The model under review builds one solid part; all positions refer to its coordinate system, in mm. Face numbers are marked on the shaded views. A direction names the side the tool comes from. Coordinates: 2 decimals unless noted, no trailing zeros. Loops run counter-clockwise (first coordinate to the right, second up) from the corner with the lowest first, then second, coordinate; pieces in that order, holes last. Notation, with made-up numbers: M 23,6 L 40,6 A20 cw 40,21 Z; hole C 28,-21.75 d1. An arc over 180 degrees is marked long. Return JSON: item names as keys, results as strings.
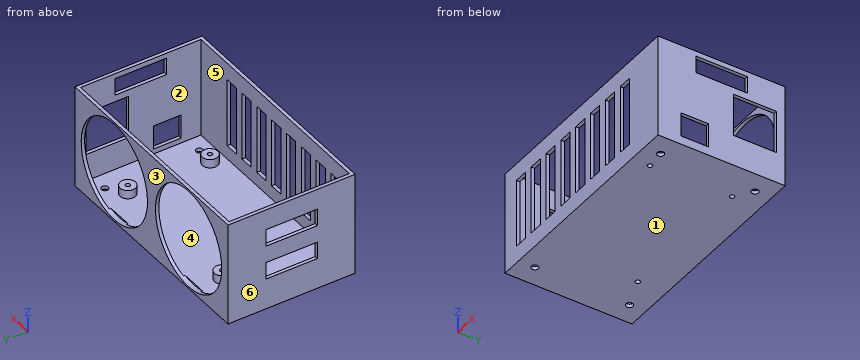
```python
from build123d import *
from build123d.topology import SkipClean

# Parameters (mm, degrees)
ESBO_O1_W                = 134
ESBO_O1_H                = 74
ESBO_O1_W_2              = 130
ESBO_O1_H_2              = 70
RESSALTO_EXTRUS_O1_DEPTH = 60
ESBO_O2_W                = 134
ESBO_O2_H                = 74
ESBO_O2_R                = 2
RESSALTO_EXTRUS_O2_DEPTH = 2
ESBO_O3_W                = 25
ESBO_O3_H                = 25
ESBO_O3_W_2              = 14
ESBO_O3_H_2              = 16
ESBO_O3_W_3              = 10
ESBO_O3_H_3              = 30
CORTE_EXTRUS_O1_DEPTH    = 10
ESBO_O6_W                = 8
ESBO_O6_H                = 40
CORTE_EXTRUS_O2_DEPTH    = 10
ESBO_O7_W                = 10
ESBO_O7_H                = 30
CORTE_EXTRUS_O3_DEPTH    = 12
ESBO_O8_R                = 4.5
ESBO_O8_R_2              = 1.35
RESSALTO_EXTRUS_O3_DEPTH = 5
ESBO_O8_3_R              = 1.35
CORTE_EXTRUS_O4_DEPTH    = 97.031244915
ESBO_O9_R                = 3
CORTE_EXTRUS_O5_DEPTH    = 2
ESBO_O10_R               = 29
CORTE_EXTRUS_O6_DEPTH    = 3


with BuildPart() as part:
    # Esboço1 → Ressalto-extrusão1 (new body)
    with BuildSketch(Plane.XY):
        Rectangle(ESBO_O1_W, ESBO_O1_H)
        Rectangle(ESBO_O1_W_2, ESBO_O1_H_2, mode=Mode.SUBTRACT)
    extrude(amount=RESSALTO_EXTRUS_O1_DEPTH)

    # Esboço2 → Ressalto-extrusão2 (add)
    with BuildSketch(Plane(origin=(0, 0, 0), x_dir=(-1, 0, 0), z_dir=(0, 0, -1))):
        Rectangle(ESBO_O2_W, ESBO_O2_H)
        with Locations((-55, -27.5)):
            Circle(ESBO_O2_R, mode=Mode.SUBTRACT)
        with Locations((55, -27.5)):
            Circle(ESBO_O2_R, mode=Mode.SUBTRACT)
        with Locations((55, 27.5)):
            Circle(ESBO_O2_R, mode=Mode.SUBTRACT)
        with Locations((-55, 27.5)):
            Circle(ESBO_O2_R, mode=Mode.SUBTRACT)
    extrude(amount=-RESSALTO_EXTRUS_O2_DEPTH)

    # Esboço3 → Corte-extrusão1 (cut)
    with BuildSketch(Plane(origin=(67, 0, 0), x_dir=(0, 0, -1), z_dir=(1, 0, 0))):
        with Locations((-30.5, 19.5)):
            Rectangle(ESBO_O3_W, ESBO_O3_H)
        with Locations((-12, -15.5)):
            Rectangle(ESBO_O3_W_2, ESBO_O3_H_2)
        with Locations((-52, 0)):
            Rectangle(ESBO_O3_W_3, ESBO_O3_H_3)
    extrude(amount=-CORTE_EXTRUS_O1_DEPTH, mode=Mode.SUBTRACT)

    # Esboço6 → Corte-extrusão2 (cut)
    with BuildSketch(Plane.XZ.offset(37)):
        with Locations((-53, 30)):
            Rectangle(ESBO_O6_W, ESBO_O6_H)
        with Locations((-40, 30)):
            Rectangle(ESBO_O6_W, ESBO_O6_H)
        with Locations((-27, 30)):
            Rectangle(ESBO_O6_W, ESBO_O6_H)
        with Locations((-14, 30)):
            Rectangle(ESBO_O6_W, ESBO_O6_H)
        with Locations((-1, 30)):
            Rectangle(ESBO_O6_W, ESBO_O6_H)
        with Locations((12, 30)):
            Rectangle(ESBO_O6_W, ESBO_O6_H)
        with Locations((25, 30)):
            Rectangle(ESBO_O6_W, ESBO_O6_H)
        with Locations((38, 30)):
            Rectangle(ESBO_O6_W, ESBO_O6_H)
    extrude(amount=-CORTE_EXTRUS_O2_DEPTH, mode=Mode.SUBTRACT)

    # Esboço7 → Corte-extrusão3 (cut)
    with BuildSketch(Plane.ZY.offset(67)):
        with Locations((43, 0)):
            Rectangle(ESBO_O7_W, ESBO_O7_H)
        with Locations((23, 0)):
            Rectangle(ESBO_O7_W, ESBO_O7_H)
    extrude(amount=-CORTE_EXTRUS_O3_DEPTH, mode=Mode.SUBTRACT)

    # Esboço8 → Ressalto-extrusão3 (add)
    # profile 1 of 3: a face of its own
    with BuildSketch(Plane(origin=(0, 0, 2), x_dir=(-1, 0, 0), z_dir=(0, 0, -1))):
        with Locations(Location((37.05, 20.5, 0), (0, 0, 180))):
            Circle(ESBO_O8_R)
        with Locations(Location((37.05, 20.5, 0), (0, 0, 180))):
            Circle(ESBO_O8_R_2, mode=Mode.SUBTRACT)
    # profile 2 of 3: a face of its own
    with BuildSketch(Plane(origin=(0, 0, 2), x_dir=(-1, 0, 0), z_dir=(0, 0, -1))):
        with Locations(Location((-45.5, 20.5, 0), (0, 0, 180))):
            Circle(ESBO_O8_R)
        with Locations(Location((-45.5, 20.5, 0), (0, 0, 180))):
            Circle(ESBO_O8_R_2, mode=Mode.SUBTRACT)
    # profile 3 of 3: a face of its own
    with BuildSketch(Plane(origin=(0, 0, 2), x_dir=(-1, 0, 0), z_dir=(0, 0, -1))):
        with Locations(Location((-44.2, -26.5, 0), (0, 0, 180))):
            Circle(ESBO_O8_R)
        with Locations(Location((-44.2, -26.5, 0), (0, 0, 180))):
            Circle(ESBO_O8_R_2, mode=Mode.SUBTRACT)
    extrude(amount=-RESSALTO_EXTRUS_O3_DEPTH)

    # Esboço8<3> → Corte-extrusão4 (cut, through all)
    with SkipClean():  # the faces are left unmerged after this step: merging them gives an invalid solid
        with BuildSketch(Plane(origin=(0, 0, 2), x_dir=(-1, 0, 0), z_dir=(0, 0, -1))):
            with Locations((-44.2, -26.5)):
                Circle(ESBO_O8_3_R)
            with Locations((37.05, 20.5)):
                Circle(ESBO_O8_3_R)
            with Locations((-45.5, 20.5)):
                Circle(ESBO_O8_3_R)
        extrude(amount=CORTE_EXTRUS_O4_DEPTH, mode=Mode.SUBTRACT)

    # Esboço9 → Corte-extrusão5 (cut)
    with BuildSketch(Plane.XY.offset(2)):
        with Locations((45.5, 20.5)):
            Circle(ESBO_O9_R)
        with Locations((44.2, -26.5)):
            Circle(ESBO_O9_R)
        with Locations((-37.05, 20.5)):
            Circle(ESBO_O9_R)
    extrude(amount=CORTE_EXTRUS_O5_DEPTH, mode=Mode.SUBTRACT)

    # Esboço10 → Corte-extrusão6 (cut)
    with BuildSketch(Plane(origin=(0, 37, 0), x_dir=(1, 0, 0), z_dir=(0, 1, 0))):
        with Locations(Location((32.5, -30, 0), (0, 0, 270))):
            Circle(ESBO_O10_R)
        with Locations(Location((-32.5, -30, 0), (0, 0, 270))):
            Circle(ESBO_O10_R)
    extrude(amount=-CORTE_EXTRUS_O6_DEPTH, mode=Mode.SUBTRACT)


solid = part.part
```
1. Add section A-A on x = 1. Give the boundary of the cut face in (y, z), plus the area to 3 significant figures.
Check values:
{"outline": "M -37,0 L 37,0 L 37,60 L 35,60 L 35,2 L -35,2 L -35,10 L -37,10 Z; M -37,50 L -35,50 L -35,60 L -37,60 Z", "area": "300 mm²"}
2. Add section D-D on z = 53. Give the boundary of the cut face in (x, y).
Check values:
{"outline": "M -67,-37 L 67,-37 L 67,-15 L 65,-15 L 65,-35 L -65,-35 L -65,35 L -50.16,35 L -50.16,37 L -67,37 Z; M -14.84,35 L 14.84,35 L 14.84,37 L -14.84,37 Z; M 50.16,35 L 65,35 L 65,15 L 67,15 L 67,37 L 50.16,37 Z"}
3. Add section C-C on y = -17.5. Give the boundary of the cut face in (x, z), plus the area to 3 significant figures.
Check values:
{"outline": "M -67,0 L 67,0 L 67,5 L 65,5 L 65,2 L -65,2 L -65,60 L -67,60 Z; M 65,19 L 67,19 L 67,60 L 65,60 Z", "area": "472 mm²"}
4. The part is to be moulded in two halves that separate along X. For the marked faces 3, 4, 5 and 6, say which applies: released by +X, released by -X, zero draft, split by the parting line, or undercut.
Check values:
{"face 3": "zero draft", "face 4": "undercut", "face 5": "undercut", "face 6": "released by -X"}
5. Add section B-B on y = 27.5. Give the boundary of the cut face in (x, z).
Check values:
{"outline": "M -67,0 L -57,0 L -57,2 L -65,2 L -65,60 L -67,60 Z; M -53,0 L 53,0 L 53,2 L -53,2 Z; M 57,0 L 67,0 L 67,18 L 65,18 L 65,2 L 57,2 Z; M 65,43 L 67,43 L 67,60 L 65,60 Z"}
6. Insertion check: pin 1 Ø2 at (x, y) = (26.5, -36) entering from -Z; pin 2 Ø1 at (y, z) = (24, 38) entering from +X; pin 3 Ø7 at (x, y) = (43, -27.5) entering from +Z; pin 4 Ø6 at (x, z) = (21.5, 31.5) entering from +Y. Each pin has a flat end and moves straight along its axis. Give the tip position at first contact, or say it passes through.
Check values:
{"pin 1": "z = 0", "pin 2": "x = -65", "pin 3": "z = 7", "pin 4": "y = -35"}
7. To check wall thickness, follow line 1 (Y direction, x = -55, z = 0.6); line 2 (X direction, y = 20.5, z = 0.85); line 3 (X direction, y = -5.5, z = 10.5). State the ranges of each line that lie inside material, in increasing order.
Check values:
{"line 1": "-37 to -29.5, -25.5 to 25.5, 29.5 to 37", "line 2": "-67 to -38.4, -35.7 to 44.15, 46.85 to 67", "line 3": "-67 to -65, 65 to 67"}
8. Machinability: for the marked faces 1 and 2, which of the approach directions +Z, -Z, +X, -X, +Y, -Y give a long, thin tool a straight path to every point of the face, cutting with its end or side? Answer none if there is none.
Check values:
{"face 1": "-Z, +X, -X, +Y, -Y", "face 2": "+Z"}
